```python
from build123d import *

# Parameters (mm, degrees)
SKETCH1_W                 = 14
SKETCH1_H                 = 5
BOSS_EXTRUDE1_DEPTH       = 18
SKETCH2_W                 = 12
SKETCH2_H                 = 3
CUT_EXTRUDE1_DEPTH        = 8
F_8_CLEARANCE_HOLE1_D     = 4.4958
F_8_CLEARANCE_HOLE1_DEPTH = 17
F_8_CLEARANCE_HOLE1_TIP   = 1.350674586


with BuildPart() as part:
    # Sketch1 → Boss-Extrude1 (new body)
    with BuildSketch(Plane.XY):
        with Locations((2.953810723, -0.588235294)):
            Rectangle(SKETCH1_W, SKETCH1_H)
    extrude(amount=-BOSS_EXTRUDE1_DEPTH)

    # Sketch2 → Cut-Extrude1 (cut)
    with BuildSketch(Plane.XY):
        with Locations((2.953810723, -0.588235294)):
            Rectangle(SKETCH2_W, SKETCH2_H)
    extrude(amount=-CUT_EXTRUDE1_DEPTH, mode=Mode.SUBTRACT)

    # #8 Clearance Hole1
    with Locations(Plane(origin=(2.953810723, -3.088235294, -15), x_dir=(0, 0, -1), z_dir=(0, -1, 0))):
        with Locations((0, 0)):
            Hole(F_8_CLEARANCE_HOLE1_D / 2, depth=F_8_CLEARANCE_HOLE1_DEPTH)
            with Locations((0, 0, -(F_8_CLEARANCE_HOLE1_DEPTH + F_8_CLEARANCE_HOLE1_TIP / 2))):  # 118° drill point
                Cone(0, F_8_CLEARANCE_HOLE1_D / 2, F_8_CLEARANCE_HOLE1_TIP, mode=Mode.SUBTRACT)


solid = part.part
```
The model under review builds one solid part; all positions refer to its coordinate system, in mm. A direction names the side the tool comes from. Round coordinates to 2 decimals unless told otherwise and drop trailing zeros. Order: outer loops, then holes, each group sorted by start corner. A loop starts at its lowest first (then second) coordinate and runs counter-clockwise, first axis right, second up. Notation, with made-up numbers: (83.25, -35) - (99.25, -35) arc R18 ccw to (99.25, -3) - close; hole circle Ø5 at (-30, 26.5). An arc over 180 degrees is marked (long way). Answer in a Markdown table with one row per item.
(1) Take a section at C-C on z = -2.25. Write out the cut boundary in (x, y), plus the area to 3 significant figures.
Result set:
| item | result |
|---|---|
| outline | (-4.05, -3.09) - (9.95, -3.09) - (9.95, 1.91) - (-4.05, 1.91) - close; hole (-3.05, -2.09) - (8.95, -2.09) - (8.95, 0.91) - (-3.05, 0.91) - close |
| area | 34.0 mm2 |
(2) Take a section at D-D on x = 3.5. Write out the cut boundary in (y, z).
Result set:
| item | result |
|---|---|
| outline | (-3.09, -18) - (1.91, -18) - (1.91, -17.18) - (-3.09, -17.18) - close; (-3.09, -12.82) - (1.91, -12.82) - (1.91, 0) - (0.91, 0) - (0.91, -8) - (-2.09, -8) - (-2.09, 0) - (-3.09, 0) - close |
(3) Clearance check with flat-ended pins moving along their axes: P1, Ø4, axis at x = 2.95, z = -15, coming from the +Y side; P2, Ø2, axis at x = 1.5, y = -0.5, coming from the +Z side. State where each tip first meets the part, or that it passes through.
Result set:
| item | result |
|---|---|
| P1 | passes through |
| P2 | stops at z = -8 |
(4) Mouldability with a two-part tool opening along Y and no side actions: class faces 3 (the face through (-3.046, -1, -4)), 4 (the face through (3, 1.912, -9)), 5 (the face through (3, -2.088, -4)), 6 (the face through (3.629, -0.553, -12.856)) as released by +Y, released by -Y, zero draft, split by the parting line, or undercut.
Result set:
| item | result |
|---|---|
| face 3 | undercut |
| face 4 | released by +Y |
| face 5 | undercut |
| face 6 | zero draft |
(5) Take a section at A-A on z = -15. Write out the cut boundary in (x, y), plus the area to 3 significant figures.
Result set:
| item | result |
|---|---|
| outline | (-4.05, -3.09) - (0.71, -3.09) - (0.71, 1.91) - (-4.05, 1.91) - close; (5.2, -3.09) - (9.95, -3.09) - (9.95, 1.91) - (5.2, 1.91) - close |
| area | 47.5 mm2 |
(6) For line 1 (X direction, y = -0.65, z = -15); line 2 (Y direction, x = 2, z = -2); line 3 (X direction, y = -0.45, z = -1), list the stretches that pass through material, from the lowest coordinate up. Write a range as from..to.
Result set:
| item | result |
|---|---|
| line 1 | x = -4.05..0.71, 5.2..9.95 |
| line 2 | y = -3.09..-2.09, 0.91..1.91 |
| line 3 | x = -4.05..-3.05, 8.95..9.95 |
(7) Machinability: for faces 1 (the face through (-4.046, -1, -9)), 2 (the face through (8.954, -1, -4)), which of the approach directions +Z, -Z, +X, -X, +Y, -Y give a long, thin tool a straight path to every point of the face, cutting with its end or side? Answer none if there is none.
Result set:
| item | result |
|---|---|
| face 1 | +Z, -Z, -X, +Y, -Y |
| face 2 | +Z |
(8) Take a section at B-B on x = -0.5. Write out the cut boundary in (y, z).
Result set:
| item | result |
|---|---|
| outline | (-3.09, -18) - (1.91, -18) - (1.91, 0) - (0.91, 0) - (0.91, -8) - (-2.09, -8) - (-2.09, 0) - (-3.09, 0) - close |
